Can you work these out from the model? Positions are in its coordinate system, mm. Face numbers are marked on the shaded views. A direction names the side the tool comes from. Give positions to 0.01 mm unless a question says otherwise; leave off trailing zeros. Loops run counter-clockwise (first coordinate to the right, second up) from the corner with the lowest first, then second, coordinate; pieces in that order, holes last.
from build123d import *

# Parameters (mm, degrees)
SCHNITT_LINEAR_AUSTRAGEN1_DEPTH      = 3
SCHNITT_LINEAR_AUSTRAGEN1_DEPTH_BACK = 3


with BuildPart() as part:
    # Skizze1 → Rotation1 (revolve)
    with BuildSketch(Plane(origin=(0, 0, 0), x_dir=(1, 0, 0), z_dir=(0, 1, 0))):
        with BuildLine():
            Line((0, 0), (-2.9, 0))
            Line((-2.9, 0), (-2.9, 5.859069893))
            ThreePointArc((-2.9, 5.859069893), (-3.518262416, 6.494321905), (-4, 7.238447187))
            Line((-4, 7.238447187), (-4, 11.361552813))
            ThreePointArc((-4, 11.361552813), (-3.626876384, 11.963788222), (-3.163858404, 12.5))
            Line((-3.163858404, 12.5), (0, 12.5))
            Line((0, 12.5), (0, 0))
        make_face()
    revolve(axis=Axis((0, 0, -12.5), (0, 0, 1)))

    # Skizze2 → Schnitt-Linear austragen1 (cut, two sides)
    with BuildSketch(Plane.XY) as schnitt_linear_austragen1_sk:
        Polygon((6, 4), (2.5, 4), (2.5, -5), (-2.5, -5), (-2.5, 4), (-6, 4), (-6, -6), (6, -6), align=None)
    extrude(amount=SCHNITT_LINEAR_AUSTRAGEN1_DEPTH, mode=Mode.SUBTRACT)
    extrude(schnitt_linear_austragen1_sk.sketch, amount=-SCHNITT_LINEAR_AUSTRAGEN1_DEPTH_BACK, mode=Mode.SUBTRACT)

    # Skizze3 → Rotation2 (revolve)
    with BuildSketch(Plane(origin=(0, 0, 0), x_dir=(1, 0, 0), z_dir=(0, 1, 0))):
        Polygon((0, -12), (-2.3865, -12), (-3, -11.3865), (-3, -1.5), (-2.454044649, 0), (0, 0), align=None)
    revolve(axis=Axis((0, 0, 0), (0, 0, 1)))


solid = part.part
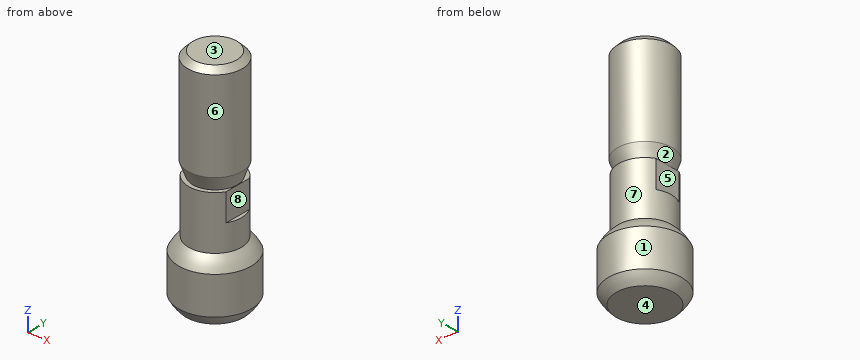
(1) Thinking about a two-plate mould opening in Z: for the marked faces 1, 2 and 3, which applies, pulls with the +Z half, pulls with the -Z half, needs draft (parallel to the pull), parting line crosses it, or undercut?
Returned:
face 1: needs draft
face 2: undercut
face 3: pulls with the +Z half
(2) Which directions (+Z, -Z, +X, -X, +Y, -Y) give clear straight access to the entire face, cutting with the end or side of a thin tool? Please do the marked faces 4, 5, 6, 7 and 8.
Returned:
face 4: -Z, +X, -X, +Y, -Y
face 5: -X, +Y, -Y
face 6: +Z
face 7: none
face 8: +X, +Y, -Y
(3) Please list where these lines run through material, in increasing order: probe 1 along Y at (x, z) = (2.5, -3.25); probe 2 along X at (y, z) = (-1.5, -8); probe 3 along Z at (x, y) = (2.25, -3).
Returned:
probe 1: y = -1.47 to 1.47
probe 2: x = -3.71 to 3.71
probe 3: z = -11.79 to -6.81
(4) Suppose I cut it at A-A on x = 0. List the corners of the cut face in (y, z) for me.
Returned:
outline: (-4, -11.36) arc R4.5 ccw to (-3.16, -12.5) - (3.16, -12.5) arc R4.5 ccw to (4, -11.36) - (4, -7.24) arc R4.5 ccw to (2.9, -5.86) - (2.9, 0) - (2.45, 0) - (3, 1.5) - (3, 11.39) - (2.39, 12) - (-2.39, 12) - (-3, 11.39) - (-3, 1.5) - (-2.45, 0) - (-2.9, 0) - (-2.9, -5.86) arc R4.5 ccw to (-4, -7.24) - close
(5) Suppose I cut it at C-C on z = -7.5. List the corners of the cut face in (x, y) for me.
Returned:
outline: circle Ø8 at (0, 0)
(6) Will these pins go through, and if not, where does the flat tip stop? P1, Ø0.9, axis at y = 0.5, z = -2, coming from the +X side; P2, Ø1, axis at y = -1.5, z = 2, coming from the +X side.
Returned:
P1: stops at x = 2.5
P2: stops at x = 2.83
(7) Suppose I cut it at B-B on z = 10.25. List the corners of the cut face in (x, y) for me.
Returned:
outline: circle Ø6 at (0, 0)
(8) Suppose I cut it at D-D on z = -0.5. List the corners of the cut face in (x, y) for me, plus the area to 3 significant figures.
Returned:
outline: (-2.5, -1.47) arc R2.9 ccw to (2.5, -1.47) - (2.5, 1.47) arc R2.9 ccw to (-2.5, 1.47) - close
area: 24.8 mm2
